Work out the finished part from the listing and answer in its coordinate system (mm). Face numbers are marked on the shaded views. A direction names the side the tool comes from. Coordinates: 2 decimals unless noted, no trailing zeros. Order: outer loops, then holes, each group sorted by start corner. A loop starts at its lowest first (then second) coordinate and runs counter-clockwise, first axis right, second up. Notation, with made-up numbers: M 41,-36 L 79,-36 A20 cw 79,-32 Z; hole C -16,66 d1. An arc over 180 degrees is marked long. Use a Markdown table: item, result.
from build123d import *

# Parameters (mm, degrees)
SKETCH1_W           = 11.8
SKETCH1_H           = 1.5
BOSS_EXTRUDE1_DEPTH = 20
SKETCH3_W           = 25
SKETCH3_H           = 25
SKETCH3_R           = 1.4
BOSS_EXTRUDE2_DEPTH = 5
SKETCH4_R           = 1.6
CUT_EXTRUDE2_DEPTH  = 7.5


with BuildPart() as part:
    # Sketch1 → Boss-Extrude1 (new body)
    with BuildSketch(Plane.XY):
        Polygon((-6.6, 1.5), (0, 1.5), (11.8, 1.5), (18.4, 1.5), (18.4, 6.5), (-6.6, 6.5), align=None)
        with Locations((5.9, 0.75)):
            Rectangle(SKETCH1_W, SKETCH1_H)
    extrude(amount=BOSS_EXTRUDE1_DEPTH)

    # Sketch3 → Boss-Extrude2 (add)
    with BuildSketch(Plane(origin=(0, 0, 0), x_dir=(-1, 0, 0), z_dir=(0, 0, -1))):
        with Locations((-5.9, 19)):
            Rectangle(SKETCH3_W, SKETCH3_H)
        with Locations((-5.9, 16.5)):
            Circle(SKETCH3_R, mode=Mode.SUBTRACT)
        with Locations((-5.9, 26.5)):
            Circle(SKETCH3_R, mode=Mode.SUBTRACT)
    extrude(amount=-BOSS_EXTRUDE2_DEPTH)

    # Sketch4 → Cut-Extrude2 (cut, through all)
    with BuildSketch(Plane(origin=(0, 6.5, 0), x_dir=(1, 0, 0), z_dir=(0, 1, 0))):
        with Locations((5.9, -13)):
            Circle(SKETCH4_R)
    extrude(amount=-CUT_EXTRUDE2_DEPTH, mode=Mode.SUBTRACT)


solid = part.part
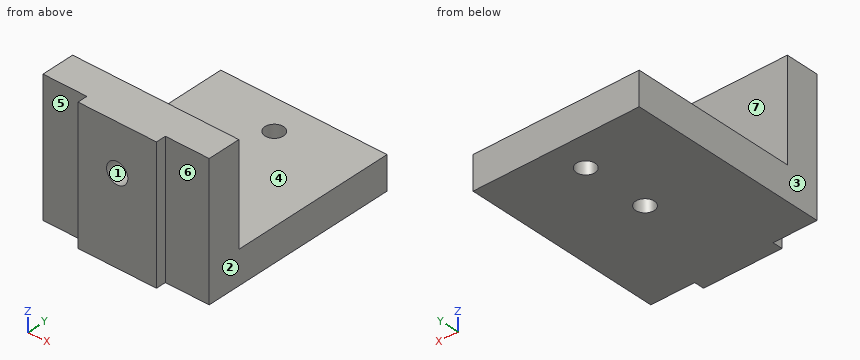
(1) Determine the mould class of the marked faces 1, 2, 3 and 4 for opening direction X: pulls with the +X half, pulls with the -X half, needs draft (parallel to the pull), parting line crosses it, or undercut.
Conclusion:
| item | result |
|---|---|
| face 1 | undercut |
| face 2 | pulls with the +X half |
| face 3 | pulls with the -X half |
| face 4 | needs draft |
(2) Which of the six approach directions +Z, -Z, +X, -X, +Y, -Y give full straight-line access (tool end or side, diameter ignored) to the marked faces 5, 6 and 7?
Conclusion:
| item | result |
|---|---|
| face 5 | +Z, -Z, -X, -Y |
| face 6 | +Z, -Z, +X, -Y |
| face 7 | +Z, +X, -X, +Y |
(3) Given P1, Ø4, axis at x = -2, y = 19.5, coming from the +Z side; P2, Ø2.5, axis at x = 5.9, y = 26.5, coming from the +Z side; P3, Ø12, axis at x = 5, z = 15, coming from the +Y side; P4, Ø2, axis at x = -2, z = 6, coming from the -Y side, each flat-ended and moving along its own axis, determine where each tip first touches the part or whether it passes through.
Conclusion:
| item | result |
|---|---|
| P1 | z = 5 |
| P2 | through |
| P3 | y = 6.5 |
| P4 | y = 1.5 |
(4) A cutting plane is placed at C-C (z = 4.25). Determine the outline of the cut face in (x, y).
Conclusion:
| item | result |
|---|---|
| outline | M -6.6,1.5 L 0,1.5 L 0,0 L 11.8,0 L 11.8,1.5 L 18.4,1.5 L 18.4,31.5 L -6.6,31.5 Z; hole C 5.9,16.5 d2.8; hole C 5.9,26.5 d2.8 |
(5) A cutting plane is placed at D-D (x = 2). Determine the outline of the cut face in (y, z), then the cut area to 3 significant figures.
Conclusion:
| item | result |
|---|---|
| outline | M 0,0 L 31.5,0 L 31.5,5 L 6.5,5 L 6.5,20 L 0,20 Z |
| area | 255 mm2 |
(6) A cutting plane is placed at B-B (x = 5.9). Determine the outline of the cut face in (y, z), then the cut area to 3 significant figures.
Conclusion:
| item | result |
|---|---|
| outline | M 0,0 L 15.1,0 L 15.1,5 L 6.5,5 L 6.5,11.4 L 0,11.4 Z; M 0,14.6 L 6.5,14.6 L 6.5,20 L 0,20 Z; M 17.9,0 L 25.1,0 L 25.1,5 L 17.9,5 Z; M 27.9,0 L 31.5,0 L 31.5,5 L 27.9,5 Z |
| area | 206 mm2 |
(7) Straight lines are drawn through the part: L1, parallel to Y at x = 5.9, z = 1.1; L2, parallel to Y at x = 11, z = 19; L3, parallel to Y at x = -1, z = 16.5. For each, find the intervals that lie inside material, in ascending order.
Conclusion:
| item | result |
|---|---|
| L1 | 0 to 15.1, 17.9 to 25.1, 27.9 to 31.5 |
| L2 | 0 to 6.5 |
| L3 | 1.5 to 6.5 |
(8) A cutting plane is placed at A-A (y = 16.5). Determine the outline of the cut face in (x, z).
Conclusion:
| item | result |
|---|---|
| outline | M -6.6,0 L 4.5,0 L 4.5,5 L -6.6,5 Z; M 7.3,0 L 18.4,0 L 18.4,5 L 7.3,5 Z |
